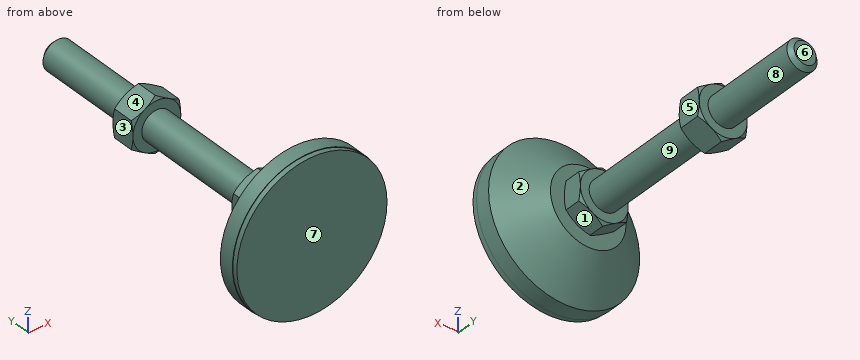
from build123d import *

# Parameters (mm, degrees)
EXTRUDE_1_DEPTH = 8
EXTRUDE_2_DEPTH = 10


with BuildPart() as part:
    # Эскиз1 → Повернуть1 (revolve)
    with BuildSketch(Plane.XY, mode=Mode.PRIVATE) as revolve_1_sk:
        Polygon((0, 0), (-29.8, 0), (-29.8, 2), (-30, 2), (-30, 8), (-15, 20), (-6, 20), (-6, 28), (-6, 126.4), (-4.4, 128), (0, 128), align=None)
    revolve(revolve_1_sk.sketch.rotate(Axis((0, 0, 0), (0, 1, 0)), 180), axis=Axis((0, 0, 0), (0, 1, 0)))  # turned: the seam where the file's is

    # Эскиз2 → Бобышка-Вытянуть1 (add)
    with BuildSketch(Plane(origin=(0, 20, 0), x_dir=(1, 0, 0), z_dir=(0, 1, 0))):
        Polygon((0, 10.969655115), (-9.5, 5.484827557), (-9.5, -5.484827557), (0, -10.969655115), (9.5, -5.484827557), (9.5, 5.484827557), align=None)
    extrude(amount=EXTRUDE_1_DEPTH)

    # Эскиз3 → Бобышка-Вытянуть2 (add)
    with BuildSketch(Plane(origin=(0, 77.2, 0), x_dir=(1, 0, 0), z_dir=(0, 1, 0))):
        Polygon((9.5, 5.484827557), (0, 10.969655115), (-9.5, 5.484827557), (-9.5, -5.484827557), (0, -10.969655115), (9.5, -5.484827557), align=None)
    extrude(amount=EXTRUDE_2_DEPTH)

    # Эскиз4 → Вырез-Повернуть2 (revolve, cut)
    with BuildSketch(Plane.XY, mode=Mode.PRIVATE) as cut_revolve_2_sk:
        Polygon((-18.160254038, 87.2), (-9.5, 87.2), (-18.160254038, 82.2), align=None)
        Polygon((-18.160254038, 77.2), (-18.160254038, 82.2), (-9.5, 77.2), align=None)
        Polygon((-16.42820323, 28), (-16.42820323, 24), (-9.5, 28), align=None)
        Polygon((-16.42820323, 24), (-16.42820323, 20), (-9.5, 20), align=None)
    revolve(cut_revolve_2_sk.sketch.rotate(Axis((0, 128, 0), (0, -1, 0)), 180), axis=Axis((0, 128, 0), (0, -1, 0)), mode=Mode.SUBTRACT)  # turned: the seam where the file's is


solid = part.part
Part model, mm, in its own coordinate system. Face numbers are marked on the shaded views. A direction names the side the tool comes from. Coordinates: 2 decimals unless noted, no trailing zeros. Write each loop counter-clockwise with the first axis right and the second up, starting at its lowest first coordinate (ties: lowest second). Pieces come first, ordered by that corner, then holes. Notation, with made-up numbers: M 3.25,-9.5 L 39.25,-9.5 A11 ccw 39.25,-2.5 Z; hole C 1.5,-21 d6. An arc over 180 degrees is marked long. Return JSON: item names as keys, results as strings.
1. Pull direction Y, two halves, no side cores. Call the marked faces 6, 7, 8 and 9: pulls with the +Y half, pulls with the -Y half, needs draft (parallel to the pull), parting line crosses it, or undercut.
Determined:
{"face 6": "pulls with the +Y half", "face 7": "pulls with the -Y half", "face 8": "needs draft", "face 9": "undercut"}
2. Flat gauge pins, fed straight in: pin 1 Ø4 at (x, y) = (2.5, 44.5) entering from -Z; pin 2 Ø4 at (x, y) = (-13, 78) entering from -Z; pin 3 Ø8 at (y, z) = (83, 2.5) entering from +X; pin 4 Ø2.5 at (y, z) = (25.5, -2) entering from -X. Where does each tip first touch, or does it go through?
Determined:
{"pin 1": "z = -5.98", "pin 2": "through", "pin 3": "x = 9.5", "pin 4": "x = -9.5"}
3. 3-axis set-ups, long thin cutter, end or side, ignore diameter. For the marked faces 1, 2, 3, 4 and 5: which of +Z, -Z, +X, -X, +Y, -Y reach the whole face in a straight line?
Determined:
{"face 1": "-Z, +X, +Y", "face 2": "+Y", "face 3": "+Z, -Z, -X, +Y", "face 4": "+Z, -X, +Y", "face 5": "+Z, -Z, +X, +Y"}
4. Probe L1, parallel to Y at x = -8, z = -12.5; L2, parallel to Z at x = -0.5, y = 67; L3, parallel to X at y = 89.5, z = -5. List the from-to ranges inside material, lowest first.
Determined:
{"L1": "0 to 20", "L2": "-5.98 to 5.98", "L3": "-3.32 to 3.32"}
5. Saw through at A-A, the plane y = 80. Write the cut outline in (x, z), then the cut area to 3 significant figures.
Determined:
{"outline": "M -9.5,-5.48 L 0,-10.97 L 9.5,-5.48 L 9.5,5.48 L 0,10.97 L -9.5,5.48 Z", "area": "313 mm²"}
